```python
from build123d import *

# Parameters (mm, degrees)
SKETCH2_W           = 74.67
SKETCH2_H           = 84.05
SKETCH2_R           = 1.7
SKETCH2_W_2         = 9.25
SKETCH2_H_2         = 9.25
SKETCH2_W_3         = 17.5
SKETCH2_H_3         = 4
SKETCH2_W_4         = 4
SKETCH2_H_4         = 5
SKETCH2_R_2         = 2.75
BOSS_EXTRUDE1_DEPTH = 4
SKETCH2_3_W         = 17.5
SKETCH2_3_H         = 4
SKETCH2_3_W_2       = 4
SKETCH2_3_H_2       = 5
BOSS_EXTRUDE2_DEPTH = 15


with BuildPart() as part:
    # Sketch2 → Boss-Extrude1 (new body)
    # profile 1 of 10: a face of its own
    with BuildSketch(Plane.XY):
        Rectangle(SKETCH2_W, SKETCH2_H)
        with Locations((-29.99, -34.68)):
            Circle(SKETCH2_R, mode=Mode.SUBTRACT)
        with Locations((29.99, -34.68)):
            Circle(SKETCH2_R, mode=Mode.SUBTRACT)
        with Locations((-29.99, 34.68)):
            Circle(SKETCH2_R, mode=Mode.SUBTRACT)
        Polygon((19.63, -19.63), (14.5, -19.63), (14.5, -23.63), (-3, -23.63), (-3, -19.63), (-19.63, -19.63), (-19.63, -14.5), (-23.63, -14.5), (-23.63, -10.5), (-19.63, -10.5), (-19.63, 10.5), (-23.63, 10.5), (-23.63, 14.5), (-19.63, 14.5), (-19.63, 19.63), (-3, 19.63), (-3, 23.63), (14.5, 23.63), (14.5, 19.63), (19.63, 19.63), (19.63, 14.5), (23.63, 14.5), (23.63, 9.5), (19.63, 9.5), (19.63, -9.5), (23.63, -9.5), (23.63, -14.5), (19.63, -14.5), align=None, mode=Mode.SUBTRACT)
        with Locations((29.99, 34.68)):
            Rectangle(SKETCH2_W_2, SKETCH2_H_2, mode=Mode.SUBTRACT)
    # profile 2 of 10: a face of its own
    with BuildSketch(Plane.XY):
        with Locations((5.75, -21.63)):
            Rectangle(SKETCH2_W_3, SKETCH2_H_3)
    # profile 3 of 10: a face of its own
    with BuildSketch(Plane.XY):
        with Locations((21.63, -12)):
            Rectangle(SKETCH2_W_4, SKETCH2_H_4)
    # profile 4 of 10: a face of its own
    with BuildSketch(Plane.XY):
        Polygon((-3, -19.63), (14.5, -19.63), (19.63, -19.63), (19.63, -14.5), (19.63, -9.5), (19.63, 9.5), (19.63, 14.5), (19.63, 19.63), (14.5, 19.63), (-3, 19.63), (-19.63, 19.63), (-19.63, 14.5), (-19.63, 10.5), (-19.63, -10.5), (-19.63, -14.5), (-19.63, -19.63), align=None)
    # profile 5 of 10: a face of its own
    with BuildSketch(Plane.XY):
        with Locations((21.63, 12)):
            Rectangle(SKETCH2_W_4, SKETCH2_H_4)
    # profile 6 of 10: a face of its own
    with BuildSketch(Plane.XY):
        with Locations((5.75, 21.63)):
            Rectangle(SKETCH2_W_3, SKETCH2_H_3)
    # profile 7 of 10: a face of its own
    with BuildSketch(Plane.XY):
        with Locations((-21.63, 12.5)):
            Rectangle(SKETCH2_W_4, SKETCH2_H_3)
    # profile 8 of 10: a face of its own
    with BuildSketch(Plane.XY):
        with Locations((-21.63, -12.5)):
            Rectangle(SKETCH2_W_4, SKETCH2_H_3)
    # profile 9 of 10: a face of its own
    with BuildSketch(Plane.XY):
        with Locations((29.99, 34.68)):
            Rectangle(SKETCH2_W_2, SKETCH2_H_2)
        with Locations((29.99, 34.68)):
            Circle(SKETCH2_R_2, mode=Mode.SUBTRACT)
    # profile 10 of 10: a face of its own
    with BuildSketch(Plane.XY):
        with Locations((29.99, 34.68)):
            Circle(SKETCH2_R_2)
        with Locations((29.99, 34.68)):
            Circle(SKETCH2_R, mode=Mode.SUBTRACT)
    extrude(amount=BOSS_EXTRUDE1_DEPTH)

    # Sketch2_3 → Boss-Extrude2 (add)
    with BuildSketch(Plane.XY):
        with Locations((5.75, -21.63)):
            Rectangle(SKETCH2_3_W, SKETCH2_3_H)
        with Locations((-21.63, -12.5)):
            Rectangle(SKETCH2_3_W_2, SKETCH2_3_H)
        with Locations((5.75, 21.63)):
            Rectangle(SKETCH2_3_W, SKETCH2_3_H)
        with Locations((21.63, -12)):
            Rectangle(SKETCH2_3_W_2, SKETCH2_3_H_2)
        with Locations((-21.63, 12.5)):
            Rectangle(SKETCH2_3_W_2, SKETCH2_3_H)
        with Locations((21.63, 12)):
            Rectangle(SKETCH2_3_W_2, SKETCH2_3_H_2)
    extrude(amount=BOSS_EXTRUDE2_DEPTH)


solid = part.part
```
Input: part model. Units: mm. Frame: model coordinates. A direction names the side the tool comes from. Round coordinates to 2 decimals unless told otherwise and drop trailing zeros. Loops run counter-clockwise (first coordinate to the right, second up) from the corner with the lowest first, then second, coordinate; pieces in that order, holes last.
1) Section query B-B on x = -29.99. Return the cut outline in (y, z) (3 decimals).
Ans:
outline: (-42.025, 0) - (-36.38, 0) - (-36.38, 4) - (-42.025, 4) - close; (-32.98, 0) - (32.98, 0) - (32.98, 4) - (-32.98, 4) - close; (36.38, 0) - (42.025, 0) - (42.025, 4) - (36.38, 4) - close
2) Material intervals for line 1 (Y direction, x = -29.99, z = 3.2) (3 decimals); line 2 (Y direction, x = 1.5, z = 5.25); line 3 (Z direction, x = 23, y = 3), sorted ascending.
Ans:
line 1: y = -42.025 to -36.38, -32.98 to 32.98, 36.38 to 42.025
line 2: y = -23.63 to -19.63, 19.63 to 23.63
line 3: z = 0 to 4
3) Pull-direction query (X, two-part tool) for faces 1 (the cylindrical face through (-28.37, 35.19, 1.97)), 2 (the flat face through (6, 19.63, 9)), 3 (the flat face through (-37.335, -1, 2)); classes: released by +X, released by -X, zero draft, split by the parting line, or undercut.
Ans:
face 1: undercut
face 2: zero draft
face 3: released by -X
4) Section query A-A on z = 5. Return the cut outline in (x, y), plus the area to 3 significant figures.
Ans:
outline: (-23.63, -14.5) - (-19.63, -14.5) - (-19.63, -10.5) - (-23.63, -10.5) - close; (-23.63, 10.5) - (-19.63, 10.5) - (-19.63, 14.5) - (-23.63, 14.5) - close; (-3, -23.63) - (14.5, -23.63) - (14.5, -19.63) - (-3, -19.63) - close; (-3, 19.63) - (14.5, 19.63) - (14.5, 23.63) - (-3, 23.63) - close; (19.63, -14.5) - (23.63, -14.5) - (23.63, -9.5) - (19.63, -9.5) - close; (19.63, 9.5) - (23.63, 9.5) - (23.63, 14.5) - (19.63, 14.5) - close
area: 212 mm2
5) Section query C-C on y = -34.68. Return the cut outline in (x, z) (3 decimals), plus the area to 3 significant figures.
Ans:
outline: (-37.335, 0) - (-31.69, 0) - (-31.69, 4) - (-37.335, 4) - close; (-28.29, 0) - (28.29, 0) - (28.29, 4) - (-28.29, 4) - close; (31.69, 0) - (37.335, 0) - (37.335, 4) - (31.69, 4) - close
area: 271 mm2
6) Pin query (flat end, axial travel): pin 1 (3 mm diameter, centred on y = 12, z = 8, fed in from -X); pin 2 (3.5 mm diameter, centred on x = 4.5, z = 9.5, fed in from +Y); pin 3 (1.5 mm diameter, centred on y = -20.5, z = 5, fed in from +X). Return the tip coordinate at first contact, or that it passes through.
Ans:
pin 1: stops at x = -23.63
pin 2: stops at y = 23.63
pin 3: stops at x = 14.5
7) Section query D-D on x = 8. Return the cut outline in (y, z) (3 decimals).
Ans:
outline: (-42.025, 0) - (42.025, 0) - (42.025, 4) - (23.63, 4) - (23.63, 15) - (19.63, 15) - (19.63, 4) - (-19.63, 4) - (-19.63, 15) - (-23.63, 15) - (-23.63, 4) - (-42.025, 4) - close
8) Set-up query: faces 4 (the flat face through (19.63, 12, 9)), 5 (the flat face through (22, 14.5, 9)), 6 (the flat face through (6, -19.63, 9)), 7 (the flat face through (-3, -22, 9)). Return all of +Z, -Z, +X, -X, +Y, -Y with unobstructed straight access to the full face (end or side cutting, diameter ignored); none if empty.
Ans:
face 4: +Z, +Y, -Y
face 5: +Z, +X, -X, +Y
face 6: +Z, +X, -X
face 7: +Z, -X, +Y, -Y
